Part print with two shaded views. Sizes in mm from the minimum x, y, z corner. Round coordinates to 2 decimals unless told otherwise and drop trailing zeros. Order: outer loops, then holes, each group sorted by start corner. A loop starts at its lowest first (then second) coordinate and runs counter-clockwise, first axis right, second up. Notation, with made-up numbers: (-14.75, -25.5) - (29.25, -25.5) arc R12 cw to (29.25, -12.5) - close; hole circle Ø8 at (3.25, 18.5). An arc over 180 degrees is marked (long way). Use one line per item in the form item = value.
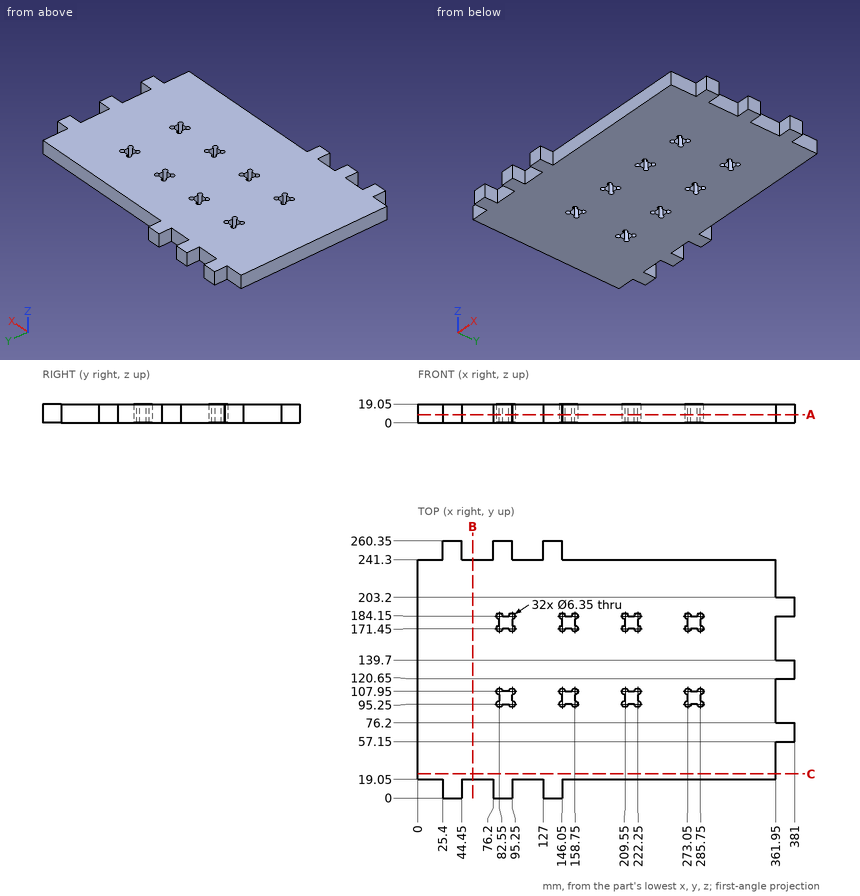
(1) Pin check, flat tips, straight feed: pin 1 (1.9 mm diameter, centred on y = 101, z = 13.5, fed in from +X); pin 2 (1.9 mm diameter, centred on x = 216, z = 10, fed in from +Y); pin 3 (3 mm diameter, centred on x = 217, z = 13.5, fed in from -Y). Stop position of each tip, or through.
Report:
pin_1 = 361.95
pin_2 = 241.3
pin_3 = 19.05
(2) Slice it at B-B on x = 55.5. Give the cut face in (y, z).
Report:
outline = (19.05, 0) - (241.3, 0) - (241.3, 19.05) - (19.05, 19.05) - close
(3) Slice it at C-C on y = 24.5. Give the cut face in (x, z), then the cut area to 3 significant figures.
Report:
outline = (0, 0) - (361.95, 0) - (361.95, 19.05) - (0, 19.05) - close
area = 6,900 mm2
(4) Probe probe 1 along Y at (x, z) = (223, 7); probe 2 along X at (y, z) = (247, 9.5); probe 3 along X at (y, z) = (105.5, 11). List the from-to ranges inside material, lowest first. Write a range as [from, to].
Report:
probe_1 = [19.05, 92.16], [98.34, 104.86], [111.04, 168.36], [174.54, 181.06], [187.24, 241.3]
probe_2 = [25.4, 44.45], [76.2, 95.25], [127, 146.05]
probe_3 = [0, 80.53], [97.27, 144.03], [160.77, 207.53], [224.27, 271.03], [287.77, 361.95]
(5) Slice it at A-A on z = 8.25. Count the separate pieces of the cut face and the enclosed holes in it, then the cut area to 3 significant figures.
Report:
separate_pieces = 1
enclosed_holes = 8
area = 81,700 mm2
